Autodesk Inventor part; units mm, degrees
ref_plane "YZ Plane" through (0, 0, 0) normal (1, 0, 0) x (0, 1, 0)
ref_plane "XZ Plane" through (0, 0, 0) normal (0, 1, 0) x (-1, 0, 0)
ref_plane "XY Plane" through (0, 0, 0) normal (0, 0, 1) x (1, 0, 0)
sketch "Skizze1" plane through (0, 0, 0) normal (0, 1, 0) x (-1, 0, 0)
  line L0 (-27.5, 22.5) -> (27.5, 22.5)
  line L1 (27.5, 22.5) -> (27.5, -22.5)
  line L2 (27.5, -22.5) -> (-27.5, -22.5)
  line L3 (-27.5, -22.5) -> (-27.5, 22.5)
  line L4 (0, -31.5) -> (0, 31.5)
  line L5 (38.5, 0) -> (-38.5, 0)
  point P0 (0, 0)
  dimension "d0" = 55
  dimension "d1" = 45
extrude "Extrusion1" add sketch "Skizze1" along normal blind 3
sketch "Skizze2" plane through (0, 3, 0) normal (0, 1, 0) x (1, 0, 0)
  line L0 (-27.5, 22.5) -> (-27.5, -22.5)
  line L1 (27.5, -22.5) -> (27.5, 22.5)
  line L2 (-27.5, -22.5) -> (27.5, -22.5)
  line L3 (27.5, -22.5) -> (27.5, -20.5)
  line L4 (27.5, -20.5) -> (-27.5, -20.5)
  line L5 (-27.5, -20.5) -> (-27.5, -22.5)
  point P0 (0, 0)
  dimension "d4" = 2
extrude "Extrusion2" add sketch "Skizze2" along normal blind 45
sketch "Skizze3" plane through (-27.5, 0, 22.5) normal (0, 0, 1) x (1, 0, 0)
  circle A0 centre (27.5, 25) radius 11.5
  line L0 (0, 0) -> (55, 0)
  line L1 (55, 0) -> (55, 48)
  circle A1 centre (43.25, 9.25) radius 1.75
  circle A2 centre (11.75, 9.25) radius 1.75
  circle A3 centre (11.75, 40.75) radius 1.75
  circle A4 centre (43.25, 40.75) radius 1.75
  line L2 (0, 48) -> (55, 48)
  line L3 (27.5, 48) -> (27.5, 0)
  line L4 (4.6208, 25) -> (55, 25)
  dimension "d7" = 23
  dimension "d10" = 3.5
  dimension "d11" = 3.5
  dimension "d12" = 3.5
  dimension "d13" = 3.5
  dimension "d17" = 31.5
  dimension "d48" = 0
extrude "Extrusion3" cut sketch "Skizze3" against normal up to surface (2 mm away) contours L4 L3 A0 | A0 L3 L4 | L3 L4 A0 | A0 L4 L3 | A1 | A2 | A3 | A4
sketch "Skizze10" plane through (0, 3, 0) normal (0, 1, 0) x (1, 0, 0)
  line L0 (27.5, -20.5) -> (27.5, 22.5)
  line L1 (27.5, 22.5) -> (-27.5, 22.5)
  line L2 (27.5, -20.5) -> (25.5, -20.5)
  line L3 (25.5, -20.5) -> (25.5, 22.5)
  line L4 (25.5, 22.5) -> (27.5, 22.5)
  line L5 (27.5, 22.5) -> (27.5, -20.5)
  line L6 (27.5, -20.5) -> (-27.5, -20.5)
  line L7 (-27.5, 22.5) -> (-25.5, 22.5)
  line L8 (-25.5, 22.5) -> (-25.5, -20.5)
  line L9 (-25.5, -20.5) -> (-27.5, -20.5)
  line L10 (-27.5, -20.5) -> (-27.5, 22.5)
  point P0 (0, 0)
  point P1 (-27.5, -20.5)
  dimension "d43" = 2
  dimension "d44" = 2
extrude "Extrusion6" add sketch "Skizze10" along normal up to surface (45 mm away) contours L2 L3 L1 L0 | L6 L10 L1 L8
sketch "Skizze11" plane through (0, 0, 0) normal (0, -1, 0) x (1, 0, 0)
  line L0 (27.5, 22.5) -> (27.5, -22.5)
  line L1 (-27.5, 22.5) -> (27.5, 22.5)
  line L2 (27.5, -22.5) -> (-27.5, -22.5)
  line L3 (-27.5, -22.5) -> (-27.5, 22.5)
  line L4 (-27.5, 22.5) -> (27.5, 22.5)
  line L5 (27.5, 22.5) -> (27.5, -22.5)
  point P0 (0, 0)
extrude "Extrusion7" add sketch "Skizze11" along normal blind 3
sketch "Skizze12" plane through (25.5, 3, -22.5) normal (0, 0, -1) x (-1, 0, 0)
  line L0 (6, -1.5) -> (14, -1.5)
  line L1 (14, -1.5) -> (14, -4.5)
  line L2 (14, -4.5) -> (6, -4.5)
  line L3 (6, -4.5) -> (6, -1.5)
  line L4 (45, -1.5) -> (37, -1.5)
  line L5 (37, -1.5) -> (37, -4.5)
  line L6 (37, -4.5) -> (45, -4.5)
  line L7 (45, -4.5) -> (45, -1.5)
  line L8 (21.5, -1.5) -> (29.5, -1.5)
  line L9 (29.5, -1.5) -> (29.5, -4.5)
  line L10 (29.5, -4.5) -> (21.5, -4.5)
  line L11 (21.5, -4.5) -> (21.5, -1.5)
  line L12 (0, 0) -> (51, 0)
  line L13 (-2, -6) -> (-2, 45)
  line L14 (53, 45) -> (53, -6)
  point P0 (25.5, -3)
  dimension "d52" = 8
  dimension "d53" = 3
  dimension "d54" = 8
  dimension "d55" = 3
  dimension "d56" = 8
  dimension "d57" = 3
  dimension "d58" = 1.5
  dimension "d59" = 1.5
  dimension "d60" = 1.5
  dimension "d61" = 8
  dimension "d62" = 8
  dimension "d63" = 7.5
extrude "Extrusion8" cut sketch "Skizze12" against normal blind 30
properties part number "Motorhalterung_v2"
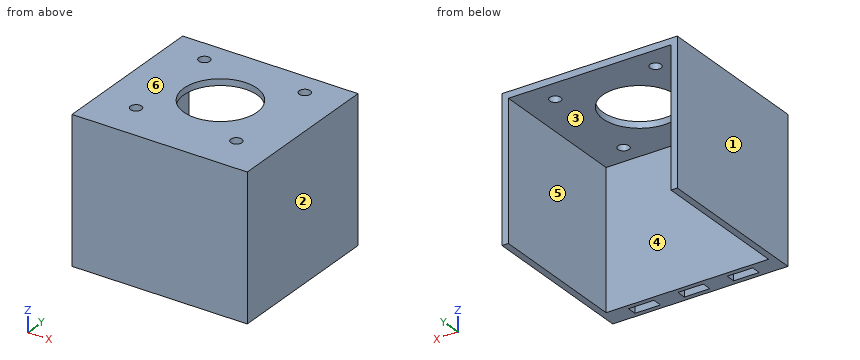
Geometry: final body of the model. Coordinates: model frame, mm. Face numbers are marked on the shaded views. A direction names the side the tool comes from. Coordinates: 2 decimals unless noted, no trailing zeros. Loops run counter-clockwise (first coordinate to the right, second up) from the corner with the lowest first, then second, coordinate; pieces in that order, holes last. Notation, with made-up numbers: M -3.75,-11 L 21.25,-11 A11 cw 21.25,-2 Z; hole C 82,63.25 d1. An arc over 180 degrees is marked long. One line per item, written item: value. Start each with the question number.
1) Material intervals for L1, parallel to X at y = 9, z = 21; L2, parallel to Y at x = -15.75, z = 21.9; L3, parallel to X at y = 8, z = -1, sorted ascending. Write a range as from..to.
2) Reachability of the marked faces 5 and 6 from +Z, -Z, +X, -X, +Y, -Y: full face, straight path, thin tool, end or side. Return the list, or none.
3) Cut plane A-A (y = 25). Return loops of the section in (x, z), then the cut area to 3 significant figures.
4) Cut plane D-D (z = 10). Return loops of the section in (x, y), then the cut area to 3 significant figures.
5) Pin query (flat end, axial travel): P1, Ø3.5, axis at x = -16, y = 0, coming from the -Z side; P2, Ø8, axis at x = -12, y = 37, coming from the -Z side; P3, Ø0.9, axis at x = 1.5, y = 0, coming from the -Z side; P4, Ø4, axis at x = -14.5, z = -6.5, coming from the +Y side. Return the tip coordinate at first contact, or that it passes through.
6) Cut plane C-C (x = 0). Return loops of the section in (y, z).
7) Draft query along X for the marked faces 1, 2, 3 and 4. Return one class per face: released by +X, released by -X, zero draft, split by the parting line, or undercut.
8) Cut plane B-B (y = 40.75). Return loops of the section in (x, z), then the cut area to 3 significant figures.
Evaluation:
1. L1: -27.5..-17.48, -14.02..14.02, 17.48..27.5
1. L2: -3..7.5, 11..39, 42.5..48
1. L3: -27.5..-25.5, 25.5..27.5
2. face 5: -Z, +Y
2. face 6: +Z, +X, -X, +Y, -Y
3. outline: M -27.5,-22.5 L -25.5,-22.5 L -25.5,20.5 L -11.5,20.5 L -11.5,22.5 L -27.5,22.5 Z; M 11.5,20.5 L 25.5,20.5 L 25.5,-22.5 L 27.5,-22.5 L 27.5,22.5 L 11.5,22.5 Z
3. area: 236 mm^2
4. outline: M -27.5,-3 L 27.5,-3 L 27.5,48 L 25.5,48 L 25.5,3 L -25.5,3 L -25.5,48 L -27.5,48 Z
4. area: 510 mm^2
5. P1: z = -22.5
5. P2: z = 20.5
5. P3: z = 7.5
5. P4: y = 3
6. outline: M -3,-22.5 L -1.5,-22.5 L -1.5,7.5 L 1.5,7.5 L 1.5,-22.5 L 3,-22.5 L 3,20.5 L 13.5,20.5 L 13.5,22.5 L -3,22.5 Z; M 36.5,20.5 L 48,20.5 L 48,22.5 L 36.5,22.5 Z
7. face 1: released by -X
7. face 2: released by +X
7. face 3: undercut
7. face 4: undercut
8. outline: M -27.5,-22.5 L -25.5,-22.5 L -25.5,20.5 L -17.5,20.5 L -17.5,22.5 L -27.5,22.5 Z; M -14,20.5 L 14,20.5 L 14,22.5 L -14,22.5 Z; M 17.5,20.5 L 25.5,20.5 L 25.5,-22.5 L 27.5,-22.5 L 27.5,22.5 L 17.5,22.5 Z
8. area: 268 mm^2
